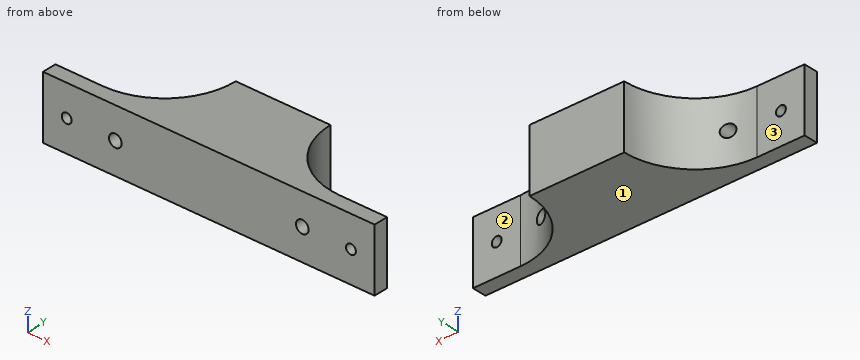
from build123d import *

# Parameters (mm, degrees)
SKETCH1_W                    = 60
SKETCH1_H                    = 40
BOSS_EXTRUDE1_DEPTH          = 54
SKETCH3_W                    = 75
SKETCH3_H                    = 40
SKETCH3_R                    = 4
BOSS_EXTRUDE2_DEPTH          = 54
CUT_EXTRUDE2_DEPTH           = 60
TAP_DRILL_FOR_M6_HELICOIL1_D = 6.25


with BuildPart() as part:
    # Sketch1 → Boss-Extrude1 (new body)
    with BuildSketch(Plane(origin=(0, 0, 0), x_dir=(1, 0, 0), z_dir=(0, 1, 0))):
        with Locations((-30, -20)):
            Rectangle(SKETCH1_W, SKETCH1_H)
    extrude(amount=BOSS_EXTRUDE1_DEPTH)

    # Sketch3 → Boss-Extrude2 (add)
    with BuildSketch(Plane(origin=(0, 0, 0), x_dir=(1, 0, 0), z_dir=(0, 1, 0))):
        with Locations((37.5, -20)):
            Rectangle(SKETCH3_W, SKETCH3_H)
        with Locations((29.2, -20)):
            Circle(SKETCH3_R, mode=Mode.SUBTRACT)
    boss_extrude2 = extrude(amount=BOSS_EXTRUDE2_DEPTH)

    # Sketch4 → Cut-Extrude2 (cut)
    with BuildSketch(Plane.XY.offset(40)):
        with BuildLine():
            ThreePointArc((75, 20.458980338), (61.05699404, 11.962243847), (45, 9))
            Line((45, 9), (75, 9))
            Line((75, 9), (75, 20.458980338))
        make_face()
        with BuildLine():
            Line((45, 9), (45, 54))
            Line((45, 54), (0, 54))
            ThreePointArc((0, 54), (13.180194847, 22.180194847), (45, 9))
        make_face()
        with BuildLine():
            Line((75, 54), (45, 54))
            Line((45, 54), (45, 9))
            ThreePointArc((45, 9), (61.05699404, 11.962243847), (75, 20.458980338))
            Line((75, 20.458980338), (75, 54))
        make_face()
    cut_extrude2 = extrude(amount=-CUT_EXTRUDE2_DEPTH, mode=Mode.SUBTRACT)

    # Tap Drill for M6 Helicoil1 (through all)
    with Locations(Plane(origin=(0, 9, 0), x_dir=(1, 0, 0), z_dir=(0, 1, 0))):
        with Locations((60, -20)):
            tap_drill_for_m6_helicoil1 = Hole(TAP_DRILL_FOR_M6_HELICOIL1_D / 2)

    # Mirror1: Boss-Extrude2, Cut-Extrude2, Tap Drill for M6 Helicoil1 across plane
    add(boss_extrude2.mirror(Plane(origin=(-30, 0, 0), x_dir=(0, 0, 1), z_dir=(1, 0, 0))))
    add(cut_extrude2.mirror(Plane(origin=(-30, 0, 0), x_dir=(0, 0, 1), z_dir=(1, 0, 0))), mode=Mode.SUBTRACT)
    add(tap_drill_for_m6_helicoil1.mirror(Plane(origin=(-30, 0, 0), x_dir=(0, 0, 1), z_dir=(1, 0, 0))), mode=Mode.SUBTRACT)


solid = part.part
For this review, take the finished solid that the model builds, in its own axes (mm). Face numbers are marked on the shaded views. A direction names the side the tool comes from. Round coordinates to 2 decimals unless told otherwise and drop trailing zeros. Order: outer loops, then holes, each group sorted by start corner. A loop starts at its lowest first (then second) coordinate and runs counter-clockwise, first axis right, second up. Notation, with made-up numbers: M 76,22 L 133,22 A33 ccw 133,59 Z; hole C 9,49.25 d2. An arc over 180 degrees is marked long. Use a Markdown table: item, result. Add a question column.
Item 1: Add section B-B, the plane y = 6. Give the boundary of the cut face in (x, z) (3 decimals), then the cut area to 3 significant figures.
Item 2: To check wall thickness, follow line 1 along Z through (x, y) = (-89.2, 8.5); line 2 along Z through (x, y) = (60, 5) (3 decimals); line 3 along Y through (x, z) = (-108.5, 34.5). State the ranges of each line that lie inside material, in increasing order.
Item 3: Add section A-A, the plane x = 60. Give the boundary of the cut face in (y, z) (3 decimals).
Item 4: Tool access review of the marked faces 1, 2 and 3: name each direction out of +Z, -Z, +X, -X, +Y, -Y from which nothing blocks a thin tool from reaching the whole face with its end or side.
Item 5: Insertion check: pin 1 (1 mm diameter, centred on y = 42, z = 4, fed in from -X); pin 2 (3 mm diameter, centred on y = 30, z = 4.5, fed in from +X); pin 3 (7 mm diameter, centred on x = -120, z = 20, fed in from +Y); pin 4 (4 mm diameter, centred on x = 60, z = 20, fed in from -Y). Each pin has a flat end and moves straight along its axis. Give the tip position at first contact, or say it passes through.
Item 6: Add section C-C, the plane z = 11. Give the boundary of the cut face in (x, y).
Item 7: Add section D-D, the plane y = 27. Give the boundary of the cut face in (x, z).
Geometry results:
| question | item | result |
|---|---|---|
| 1 | outline | M -135,0 L 75,0 L 75,40 L -135,40 Z; hole C -120,20 d6.25; hole C -89.2,20 d8; hole C 29.2,20 d8; hole C 60,20 d6.25 |
| 1 | area | 8,240 mm² |
| 2 | line 1 | z = 0 to 16, 24 to 40 |
| 2 | line 2 | z = 0 to 16.875, 23.125 to 40 |
| 2 | line 3 | y = 0 to 9 |
| 3 | outline | M 0,0 L 9,0 L 9,16.875 L 0,16.875 Z; M 0,23.125 L 9,23.125 L 9,40 L 0,40 Z |
| 4 | face 1 | -Z, +X, -X, +Y, -Y |
| 4 | face 2 | +Z, -Z, +X, +Y |
| 4 | face 3 | +Z, -Z, -X, +Y |
| 5 | pin 1 | stops at x = -61.77 |
| 5 | pin 2 | stops at x = 7.92 |
| 5 | pin 3 | stops at y = 9 |
| 5 | pin 4 | passes through |
| 6 | outline | M -135,0 L 75,0 L 75,9 L 45,9 A45 cw 0,54 L -60,54 A45 cw -105,9 L -135,9 Z |
| 7 | outline | M -69,0 L 9,0 L 9,40 L -69,40 Z |
